```python
from build123d import *

# Parameters (mm, degrees)
F0_W         = 52.5
F0_H         = 52.5
F0_W_2       = 42.5
F0_H_2       = 42.5
F1_DEPTH     = 33.02
F2_R         = 3.81
F1_FACE1_W   = 52.5
F1_FACE1_H   = 52.5
F1_FACE1_W_2 = 42.5
F1_FACE1_H_2 = 42.5
F3_DEPTH     = 8.128
F4_R         = 42.5432713814
F5_DEPTH     = 6.35
F6_SIZE      = 1.27
F7_R         = 3.81
F8_DEPTH     = 6.35
F9_SIZE      = 2.54


with BuildPart() as f1:
    # F0 (on Top) → F1 (new body)
    with BuildSketch(Plane.XY):
        Rectangle(F0_W, F0_H)
        Rectangle(F0_W_2, F0_H_2, mode=Mode.SUBTRACT)
    extrude(amount=F1_DEPTH)

    # F2 (on face) + F1_face1 (on face) → F3 (join)
    with BuildSketch(Plane(origin=(0, 0, 0), x_dir=(1, 0, 0), z_dir=(0, 0, -1))):
        Polygon((26.25, 26.25), (-26.25, 26.25), (-26.25, -26.25), (-5.715, -26.25), (-5.715, -21.25), (-21.25, -21.25), (-21.25, 21.25), (21.25, 21.25), (21.25, -21.25), (5.715, -21.25), (5.715, -26.25), (26.25, -26.25), align=None)
        with BuildLine():
            Line((-21.25, -21.25), (-5.715, -21.25))
            Line((-5.715, -21.25), (-5.715, -17.995))
            ThreePointArc((-5.715, -17.995), (-4.7850640303, -15.7499359697), (-2.54, -14.82))
            Line((-2.54, -14.82), (2.54, -14.82))
            ThreePointArc((2.54, -14.82), (4.7850640303, -15.7499359697), (5.715, -17.995))
            Line((5.715, -17.995), (5.715, -21.25))
            Line((5.715, -21.25), (21.25, -21.25))
            Line((21.25, -21.25), (21.25, 21.25))
            Line((21.25, 21.25), (-21.25, 21.25))
            Line((-21.25, 21.25), (-21.25, -21.25))
        make_face()
        Circle(F2_R, mode=Mode.SUBTRACT)
    with BuildSketch(Plane.XY.offset(33.02)):
        Rectangle(F1_FACE1_W, F1_FACE1_H)
        Rectangle(F1_FACE1_W_2, F1_FACE1_H_2, mode=Mode.SUBTRACT)
    extrude(amount=F3_DEPTH, dir=(0, 0, -1))

    # F4 (on face) → F5 (join)
    with BuildSketch(Plane(origin=(0, 0, -8.128), x_dir=(1, 0, 0), z_dir=(0, 0, -1))):
        Circle(F4_R)
    extrude(amount=F5_DEPTH)

    # F6
    f6_edges = [f1.edges().sort_by_distance(p)[0] for p in [
        (26.25, 0, 33.02),
        (0, 26.25, 33.02),
        (-26.25, 0, 33.02),
        (0, -26.25, 33.02),
    ]]
    chamfer(f6_edges, length=F6_SIZE)

    # F7 (on face) → F8 (cut, through all)
    with BuildSketch(Plane(origin=(0, 0, -8.128), x_dir=(1, 0, 0), z_dir=(0, 0, -1))):
        with Locations((0, 34.3966356907)):
            Circle(F7_R)
        with Locations((34.3966356907, 0)):
            Circle(F7_R)
        with Locations((0, -34.3966356907)):
            Circle(F7_R)
        with Locations((-34.3966356907, 0)):
            Circle(F7_R)
    extrude(amount=F8_DEPTH, mode=Mode.SUBTRACT)

    # F9
    f9_edges = [f1.edges().sort_by_distance(p)[0] for p in [
        (-42.543271, 0, -8.128),
    ]]
    chamfer(f9_edges, length=F9_SIZE)


solid = f1.part
```
Model file for the job. Use its own axes, mm. A direction names the side the tool comes from. Coordinates: 2 decimals unless noted, no trailing zeros. Order: outer loops, then holes, each group sorted by start corner. A loop starts at its lowest first (then second) coordinate and runs counter-clockwise, first axis right, second up. Notation, with made-up numbers: (44.5, -1.5) -> (97.5, -1.5) arc R20 ccw to (97.5, 17.5) -> close; hole circle Ø11 at (88.25, 62). An arc over 180 degrees is marked (long way). Answer as a JSON object with one key per item and string values. Group by question number.
1) Cut at A-A, the plane x = 0. Count the separate pieces of the cut face and the enclosed holes in it, then the cut area to 3 significant figures.
2) Pull direction Z, two halves, no side cores. Call faces 4 (the face through (-1, -1, -14.478)), 5 (the face through (-0.83, 3.72, -4.01)), 6 (the face through (0, 24, 0)): +Z half, -Z half, draft (parallel to the pull), parting line (faces both ways), or undercut.
3) Drill centre lines: L1, parallel to Y at x = 0, z = -12.5; L2, parallel to X at y = -19.5, z = 21. Where is each one in solid material? Low to high.
4) Cut at C-C, the plane z = -6. Write the cut outline in (x, y) (3 decimals).
5) Flat gauge pins, fed straight in: pin 1 (6 mm diameter, centred on x = -34.4, y = 0, fed in from +Z); pin 2 (10 mm diameter, centred on x = 13, z = 8, fed in from +Y); pin 3 (10 mm diameter, centred on x = 0, y = -34.4, fed in from +Z); pin 4 (5.5 mm diameter, centred on x = 0.5, z = -3.5, fed in from +Y). Where does each tip first touch, or does it go through?
6) Cut at D-D, the plane z = 4. Write the cut outline in (x, y), then the cut area to 3 significant figures.
7) Cut at B-B, the plane y = 0. Write the cut outline in (x, z).
8) Which spindle directions (+Z, -Z, +X, -X, +Y, -Y) get a long thin tool onto all of the face, cutting with end or side? Do faces 1 (the face through (4.76, 15.725, -4.007)), 2 (the face through (21.25, 0, 16)), 3 (the face through (-26.25, 0, 12)). Say none if no direction does.
Check values:
{
 "1": {"separate pieces": "4", "enclosed holes": "0", "area": "1,040 mm²"},
 "2": {"face 4": "-Z half", "face 5": "draft", "face 6": "undercut"},
 "3": {"L1": "y = -42.54 to -38.21, -30.59 to 30.59, 38.21 to 42.54", "L2": "x = -26.25 to -21.25, 21.25 to 26.25"},
 "4": {"outline": "(-26.25, -26.25) -> (26.25, -26.25) -> (26.25, 26.25) -> (5.715, 26.25) -> (5.715, 17.995) arc R3.175 cw to (2.54, 14.82) -> (-2.54, 14.82) arc R3.175 cw to (-5.715, 17.995) -> (-5.715, 26.25) -> (-26.25, 26.25) -> close; hole circle Ø7.62 at (0, 0)"},
 "5": {"pin 1": "passes through", "pin 2": "stops at y = 26.25", "pin 3": "stops at z = -8.13", "pin 4": "stops at y = 14.9"},
 "6": {"outline": "(-26.25, -26.25) -> (26.25, -26.25) -> (26.25, 26.25) -> (-26.25, 26.25) -> close; hole (-21.25, -21.25) -> (21.25, -21.25) -> (21.25, 21.25) -> (-21.25, 21.25) -> close", "area": "950 mm²"},
 "7": {"outline": "(-42.54, -14.48) -> (-38.21, -14.48) -> (-38.21, -8.13) -> (-40, -8.13) -> (-42.54, -10.67) -> close; (-30.59, -14.48) -> (30.59, -14.48) -> (30.59, -8.13) -> (26.25, -8.13) -> (26.25, 31.75) -> (24.98, 33.02) -> (21.25, 33.02) -> (21.25, 0) -> (3.81, 0) -> (3.81, -8.13) -> (-3.81, -8.13) -> (-3.81, 0) -> (-21.25, 0) -> (-21.25, 33.02) -> (-24.98, 33.02) -> (-26.25, 31.75) -> (-26.25, -8.13) -> (-30.59, -8.13) -> close; (38.21, -14.48) -> (42.54, -14.48) -> (42.54, -10.67) -> (40, -8.13) -> (38.21, -8.13) -> close"},
 "8": {"face 1": "+Z, +Y", "face 2": "+Z", "face 3": "+Z, -X, +Y, -Y"}
}
